Verification items for the finished model (mm, model axes). A direction names the side the tool comes from. Round coordinates to 2 decimals unless told otherwise and drop trailing zeros. Loops run counter-clockwise (first coordinate to the right, second up) from the corner with the lowest first, then second, coordinate; pieces in that order, holes last. Notation, with made-up numbers: (43, 82.25) -> (74, 82.25) arc R25 ccw to (74, 120.25) -> close; hole circle Ø1 at (44, 65.5). An arc over 180 degrees is marked (long way). Use a Markdown table: item, result. Add a question column.
```python
from build123d import *

# Parameters (mm, degrees)
SKETCH1_W           = 55
SKETCH1_H           = 45
BOSS_EXTRUDE1_DEPTH = 50
SKETCH2_W           = 45
SKETCH2_H           = 35
CUT_EXTRUDE1_DEPTH  = 45
SKETCH3_R           = 1.9
CUT_EXTRUDE2_DEPTH  = 20
SKETCH4_R           = 1.6
CUT_EXTRUDE3_DEPTH  = 10
CUT_EXTRUDE4_DEPTH  = 10
FILLET2_R           = 1
FILLET3_R           = 1


with BuildPart() as part:
    # Sketch1 → Boss-Extrude1 (new body)
    with BuildSketch(Plane(origin=(0, 0, 0), x_dir=(1, 0, 0), z_dir=(0, 1, 0))):
        with Locations((27.5, -22.5)):
            Rectangle(SKETCH1_W, SKETCH1_H)
    extrude(amount=BOSS_EXTRUDE1_DEPTH)

    # Sketch2 → Cut-Extrude1 (cut)
    with BuildSketch(Plane(origin=(0, 50, 0), x_dir=(1, 0, 0), z_dir=(0, 1, 0))):
        with Locations((27.5, -22.5)):
            Rectangle(SKETCH2_W, SKETCH2_H)
    extrude(amount=-CUT_EXTRUDE1_DEPTH, mode=Mode.SUBTRACT)

    # Sketch3 → Cut-Extrude2 (cut)
    with BuildSketch(Plane(origin=(0, 50, 0), x_dir=(1, 0, 0), z_dir=(0, 1, 0))):
        with Locations(Location((2.935211994, -2.935211994, 0), (0, 0, 270))):
            Circle(SKETCH3_R)
        with Locations(Location((52.064788006, -2.935211994, 0), (0, 0, 270))):
            Circle(SKETCH3_R)
        with Locations(Location((52.064788006, -42.064788006, 0), (0, 0, 270))):
            Circle(SKETCH3_R)
        with Locations(Location((2.935211994, -42.064788006, 0), (0, 0, 270))):
            Circle(SKETCH3_R)
    extrude(amount=-CUT_EXTRUDE2_DEPTH, mode=Mode.SUBTRACT)

    # Sketch4 → Cut-Extrude3 (cut)
    with BuildSketch(Plane(origin=(0, 5, 0), x_dir=(1, 0, 0), z_dir=(0, 1, 0))):
        with Locations(Location((13.75, -22.5, 0), (0, 0, 270))):
            Circle(SKETCH4_R)
        with Locations(Location((41.25, -22.5, 0), (0, 0, 270))):
            Circle(SKETCH4_R)
    extrude(amount=-CUT_EXTRUDE3_DEPTH, mode=Mode.SUBTRACT)

    # Sketch5 → Cut-Extrude4 (cut)
    with BuildSketch(Plane.ZY):
        Polygon((7.5, 11.987174728), (7.5, 7.5), (37.5, 7.5), (37.5, 12.5), align=None)
    extrude(amount=-CUT_EXTRUDE4_DEPTH, mode=Mode.SUBTRACT)

    # Fillet2
    fillet2_edges = [part.edges().sort_by_distance(p)[0] for p in [
        (0, 25, 0),
        (55, 25, 0),
        (55, 25, 45),
        (0, 25, 45),
    ]]
    fillet(fillet2_edges, radius=FILLET2_R)

    # Fillet3
    fillet3_edges = [part.edges().sort_by_distance(p)[0] for p in [
        (0, 12.243587364, 22.5),
        (0, 9.743587364, 7.5),
        (0, 7.5, 22.5),
        (0, 10, 37.5),
    ]]
    fillet(fillet3_edges, radius=FILLET3_R)


solid = part.part
```
1) Sectioned sample at B-B on y = 22.5. Enter the section's corners in (x, z), then the cut area to 3 significant figures.
2) Access from +Z, -Z, +X, -X, +Y, -Y to the whole of each face (thin tool, end or side, straight path). Record for faces 1 (the face through (1.779, 40.14, 1.427)), 2 (the face through (55, 25, 23)), 3 (the face through (3, 10, 37.5)).
3) Go/stop test with flat-tipped pins: pin 1 (2.5 mm diameter, centred on x = 52.06, z = 2.94, fed in from -Y); pin 2 (1.1 mm diameter, centred on x = 3, z = 42, fed in from +Y); pin 3 (1.9 mm diameter, centred on x = 13.75, z = 22.5, fed in from -Y); pin 4 (17.5 mm diameter, centred on x = 34.5, z = 20.5, fed in from +Y). Record where each tip stops, or that it passes through.
4) Thickness scan on line 1 (X direction, y = 2.3, z = 22.5); line 2 (X direction, y = 25.5, z = 9.5); line 3 (Z direction, x = 49.5, y = 38). Record the ranges inside material, lowest first.
5) Sectioned sample at C-C on y = 34.5. Enter the section's corners in (x, z).
6) Sectioned sample at A-A on x = 45. Enter the section's corners in (y, z).
7) Sectioned sample at D-D on z = 22.5. State how many separate pieces and enclosed holes the cut face has, then the cut area to 3 significant figures.
8) Release check for a two-part mould opening along Y. For faces 4 (the face through (3, 7.5, 22)), 5 (the face through (27, 50, 4)), 6 (the face through (27, 25, 45)) record: released by +Y, released by -Y, zero draft, split by the parting line, or undercut.
Geometry results:
| question | item | result |
|---|---|---|
| 1 | outline | (0, 1) arc R1 ccw to (1, 0) -> (54, 0) arc R1 ccw to (55, 1) -> (55, 44) arc R1 ccw to (54, 45) -> (1, 45) arc R1 ccw to (0, 44) -> close; hole (5, 5) -> (50, 5) -> (50, 40) -> (5, 40) -> close |
| 1 | area | 899 mm^2 |
| 2 | face 1 | +Y |
| 2 | face 2 | +Z, -Z, +X, +Y, -Y |
| 2 | face 3 | -X |
| 3 | pin 1 | y = 0 |
| 3 | pin 2 | y = 30 |
| 3 | pin 3 | through |
| 3 | pin 4 | y = 5 |
| 4 | line 1 | 0 to 12.15, 15.35 to 39.65, 42.85 to 55 |
| 4 | line 2 | 0 to 5, 50 to 55 |
| 4 | line 3 | 0 to 5, 40 to 45 |
| 5 | outline | (0, 1) arc R1 ccw to (1, 0) -> (54, 0) arc R1 ccw to (55, 1) -> (55, 44) arc R1 ccw to (54, 45) -> (1, 45) arc R1 ccw to (0, 44) -> close; hole circle Ø3.8 at (2.94, 2.94); hole circle Ø3.8 at (2.94, 42.06); hole (5, 5) -> (50, 5) -> (50, 40) -> (5, 40) -> close; hole circle Ø3.8 at (52.06, 2.94); hole circle Ø3.8 at (52.06, 42.06) |
| 6 | outline | (0, 0) -> (50, 0) -> (50, 5) -> (5, 5) -> (5, 40) -> (50, 40) -> (50, 45) -> (0, 45) -> close |
| 7 | separate pieces | 4 |
| 7 | enclosed holes | 0 |
| 7 | area | 669 mm^2 |
| 8 | face 4 | undercut |
| 8 | face 5 | released by +Y |
| 8 | face 6 | zero draft |
